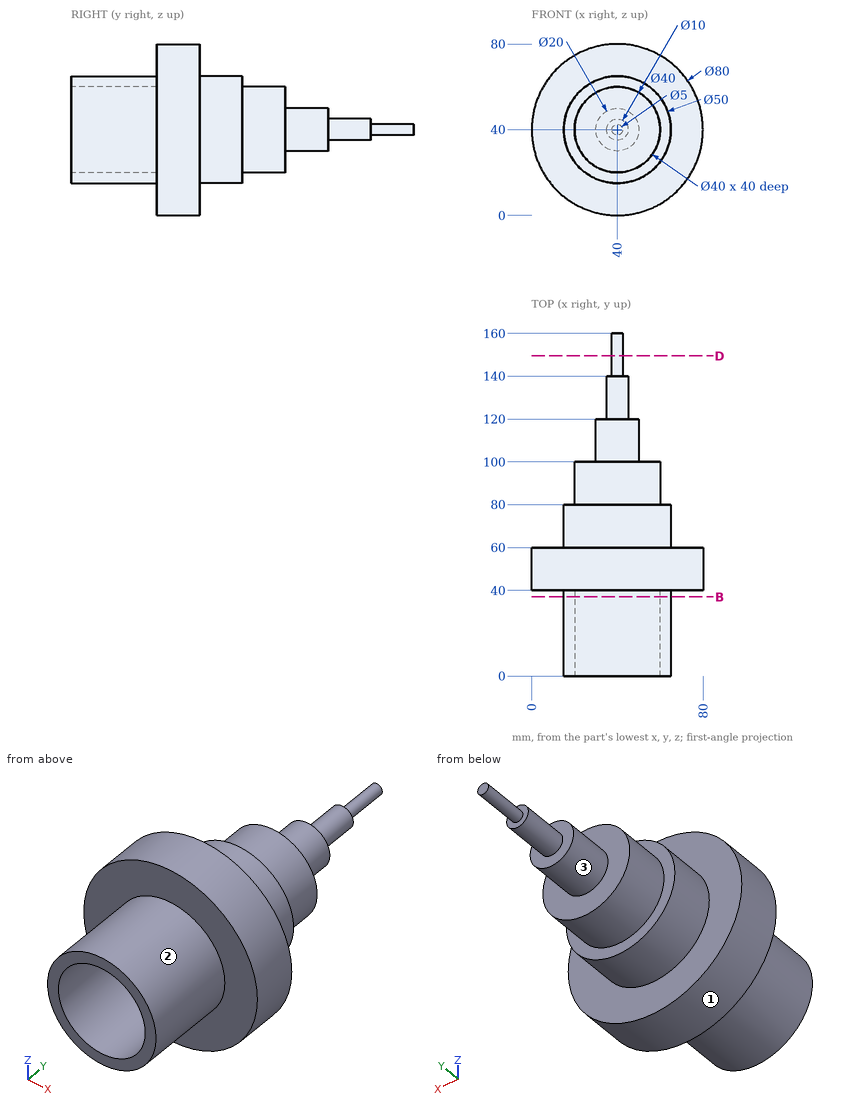
Answer from the drawing. Dimensions are ordinates in mm from the lowest x, y and z of the part. A direction names the side the tool comes from. Coordinates: 2 decimals unless noted, no trailing zeros. Write each loop counter-clockwise with the first axis right and the second up, starting at its lowest first coordinate (ties: lowest second). Pieces come first, ordered by that corner, then holes. Notation, with made-up numbers: (69, 77) - (113, 77) arc R5 ccw to (113, 84) - close; hole circle Ø7 at (-4.75, 27.25). An arc over 180 degrees is marked (long way). Return JSON: item names as keys, results as strings.
1. Each of these flat-tipped pins is pushed along its axis until it touches: pin 1 Ø8 at (x, y) = (53.5, 69.5) entering from +Z; pin 2 Ø10 at (x, y) = (32, 38.5) entering from +Z; pin 3 Ø12 at (y, z) = (122, 48.5) entering from -X; pin 4 Ø5 at (x, y) = (15.5, 84) entering from -Z. Where does it stop, or does it pass through?
Final values:
{"pin 1": "z = 63.12", "pin 2": "z = 79.87", "pin 3": "x = 30.41", "pin 4": "through"}
2. Which of the six approach directions +Z, -Z, +X, -X, +Y, -Y give full straight-line access (tool end or side, diameter ignored) to the marked faces 1, 2 and 3?
Final values:
{"face 1": "+Y, -Y", "face 2": "-Y", "face 3": "+Y"}
3. Consider line 1 along Z through (x, y) = (40, 23); line 2 along Y through (x, z) = (38.5, 58); line 3 along X through (y, z) = (38, 47.5). Determine where each line is inside the solid, lowest interval first.
Final values:
{"line 1": "15 to 20, 60 to 65", "line 2": "40 to 100", "line 3": "16.15 to 21.46, 58.54 to 63.85"}
4. The part is cut by section D-D on y = 149.5. Determine the outline of the cut face in (x, z).
Final values:
{"outline": "circle Ø5 at (40, 40)"}
5. The part is cut by section B-B on y = 37. Determine the outline of the cut face in (x, z).
Final values:
{"outline": "circle Ø50 at (40, 40); hole circle Ø40 at (40, 40)"}
